The listing builds one solid part. Answer for the finished solid, in the listing's coordinates (mm). Coordinates: 2 decimals unless noted, no trailing zeros. Order: outer loops, then holes, each group sorted by start corner. A loop starts at its lowest first (then second) coordinate and runs counter-clockwise, first axis right, second up. Notation, with made-up numbers: (35.5, 72) -> (48.5, 72) arc R4 cw to (48.5, 77) -> close; hole circle Ø1 at (86.5, -5). An arc over 180 degrees is marked (long way). Return JSON: item names as keys, results as strings.
```python
from build123d import *

# Parameters (mm, degrees)
CYLINDER021_R          = 1.5
CYLINDER021_DEPTH      = 15
CYLINDER021_ROLL_ANGLE = 90
CYLINDER020_R          = 1.5
CYLINDER020_DEPTH      = 15
CYLINDER020_ROLL_ANGLE = 90
CYLINDER018_R          = 1.5
CYLINDER018_DEPTH      = 15
CYLINDER018_ROLL_ANGLE = 90
CYLINDER019_R          = 1.5
CYLINDER019_DEPTH      = 15
CYLINDER019_ROLL_ANGLE = 90
CYLINDER017_R          = 2
CYLINDER017_DEPTH      = 25
CYLINDER016_R          = 2
CYLINDER016_DEPTH      = 25
CYLINDER001_R          = 2
CYLINDER001_DEPTH      = 25
CYLINDER002_R          = 2
CYLINDER002_DEPTH      = 25
CYLINDER003_R          = 2
CYLINDER003_DEPTH      = 25
CYLINDER_R             = 2
CYLINDER_DEPTH         = 25
BOX_W                  = 50
BOX_H                  = 100
BOX_DEPTH              = 18
CYLINDER013_R          = 2
CYLINDER013_DEPTH      = 25
CYLINDER014_R          = 2
CYLINDER014_DEPTH      = 25
CYLINDER015_R          = 2
CYLINDER015_DEPTH      = 25
CYLINDER012_R          = 2
CYLINDER012_DEPTH      = 25
BOX002_W               = 50
BOX002_H               = 100
BOX002_DEPTH           = 18
CYLINDER009_R          = 2
CYLINDER009_DEPTH      = 25
CYLINDER010_R          = 2
CYLINDER010_DEPTH      = 25
CYLINDER011_R          = 2
CYLINDER011_DEPTH      = 25
CYLINDER008_R          = 2
CYLINDER008_DEPTH      = 25
BOX003_W               = 50
BOX003_H               = 100
BOX003_DEPTH           = 18
CYLINDER005_R          = 2
CYLINDER005_DEPTH      = 25
CYLINDER006_R          = 2
CYLINDER006_DEPTH      = 25
CYLINDER007_R          = 2
CYLINDER007_DEPTH      = 25
CYLINDER004_R          = 2
CYLINDER004_DEPTH      = 25
BOX001_W               = 50
BOX001_H               = 100
BOX001_DEPTH           = 18


with BuildPart() as cilindro019:
    # Cylinder021 → Cylinder021 (new body)
    with BuildSketch(Plane.XY):
        Circle(CYLINDER021_R)
    extrude(amount=CYLINDER021_DEPTH)


with BuildPart() as cilindro019_1:
    # Cylinder021 roll: moved
    add(cilindro019.part.rotate(Axis((0, 0, 0), (1, 0, 0)), CYLINDER021_ROLL_ANGLE))


with BuildPart() as cilindro019_2:
    # Cylinder021 placement: moved
    add(cilindro019_1.part.moved(Location((20, 15, 9))))


with BuildPart() as fusion006:
    # Cylinder020 → Cylinder020 (new body)
    with BuildSketch(Plane.XY):
        Circle(CYLINDER020_R)
    extrude(amount=CYLINDER020_DEPTH)


with BuildPart() as fusion006_1:
    # Cylinder020 roll: moved
    add(fusion006.part.rotate(Axis((0, 0, 0), (1, 0, 0)), CYLINDER020_ROLL_ANGLE))


with BuildPart() as fusion006_2:
    # Cylinder020 placement: moved
    add(fusion006_1.part.moved(Location((80, 15, 9))))

    # Fusion006: union Cilindro019
    add(cilindro019_2.part)


with BuildPart() as fusion006_3:
    # Fusion006 placement: moved
    add(fusion006_2.part.moved(Location((0, 0, 4))))


with BuildPart() as mirror_of_fusion006:
    # mirror001: instance of Fusion006
    add(fusion006_3.part.mirror(Plane(origin=(0, 100, 18), x_dir=(1, 0, 0), z_dir=(0, 1, 0))))


with BuildPart() as cilindro016:
    # Cylinder018 → Cylinder018 (new body)
    with BuildSketch(Plane.XY):
        Circle(CYLINDER018_R)
    extrude(amount=CYLINDER018_DEPTH)


with BuildPart() as cilindro016_1:
    # Cylinder018 roll: moved
    add(cilindro016.part.rotate(Axis((0, 0, 0), (1, 0, 0)), CYLINDER018_ROLL_ANGLE))


with BuildPart() as cilindro016_2:
    # Cylinder018 placement: moved
    add(cilindro016_1.part.moved(Location((20, 15, 9))))


with BuildPart() as fusion005:
    # Cylinder019 → Cylinder019 (new body)
    with BuildSketch(Plane.XY):
        Circle(CYLINDER019_R)
    extrude(amount=CYLINDER019_DEPTH)


with BuildPart() as fusion005_1:
    # Cylinder019 roll: moved
    add(fusion005.part.rotate(Axis((0, 0, 0), (1, 0, 0)), CYLINDER019_ROLL_ANGLE))


with BuildPart() as fusion005_2:
    # Cylinder019 placement: moved
    add(fusion005_1.part.moved(Location((80, 15, 9))))

    # Fusion005: union Cilindro016
    add(cilindro016_2.part)


with BuildPart() as fusion005_3:
    # Fusion005 placement: moved
    add(fusion005_2.part.moved(Location((0, 0, -4))))


with BuildPart() as mirror_of_fusion005:
    # mirror: instance of Fusion005
    add(fusion005_3.part.mirror(Plane(origin=(80, 100, 18), x_dir=(-1, 0, 0), z_dir=(0, -1, 0))))


with BuildPart() as huecocentral2:
    # Cylinder017 → Cylinder017 (new body)
    with BuildSketch(Plane(origin=(50, 119, 0), x_dir=(1, 0, 0), z_dir=(0, 0, 1))):
        Circle(CYLINDER017_R)
    extrude(amount=CYLINDER017_DEPTH)


with BuildPart() as huecocentral1:
    # Cylinder016 → Cylinder016 (new body)
    with BuildSketch(Plane(origin=(50, 81, 0), x_dir=(1, 0, 0), z_dir=(0, 0, 1))):
        Circle(CYLINDER016_R)
    extrude(amount=CYLINDER016_DEPTH)


with BuildPart() as cilindro001:
    # Cylinder001 → Cylinder001 (new body)
    with BuildSketch(Plane(origin=(11, 72, 0), x_dir=(1, 0, 0), z_dir=(0, 0, 1))):
        Circle(CYLINDER001_R)
    extrude(amount=CYLINDER001_DEPTH)


with BuildPart() as cilindro002:
    # Cylinder002 → Cylinder002 (new body)
    with BuildSketch(Plane(origin=(29, 48, 0), x_dir=(1, 0, 0), z_dir=(0, 0, 1))):
        Circle(CYLINDER002_R)
    extrude(amount=CYLINDER002_DEPTH)


with BuildPart() as cilindro003:
    # Cylinder003 → Cylinder003 (new body)
    with BuildSketch(Plane(origin=(29, 72, 0), x_dir=(1, 0, 0), z_dir=(0, 0, 1))):
        Circle(CYLINDER003_R)
    extrude(amount=CYLINDER003_DEPTH)


with BuildPart() as huecos:
    # Cylinder → Cylinder (new body)
    with BuildSketch(Plane(origin=(11, 48, 0), x_dir=(1, 0, 0), z_dir=(0, 0, 1))):
        Circle(CYLINDER_R)
    extrude(amount=CYLINDER_DEPTH)

    # Fusion: union Cilindro001, Cilindro002, Cilindro003
    add(cilindro001.part)
    add(cilindro002.part)
    add(cilindro003.part)


with BuildPart() as cut003:
    # Box → Box (new body)
    with BuildSketch(Plane.XY):
        with Locations((25, 50)):
            Rectangle(BOX_W, BOX_H)
    extrude(amount=BOX_DEPTH)

    # Cut003: cut Huecos
    add(huecos.part, mode=Mode.SUBTRACT)


with BuildPart() as cilindro013:
    # Cylinder013 → Cylinder013 (new body)
    with BuildSketch(Plane(origin=(11, 72, 0), x_dir=(1, 0, 0), z_dir=(0, 0, 1))):
        Circle(CYLINDER013_R)
    extrude(amount=CYLINDER013_DEPTH)


with BuildPart() as cilindro014:
    # Cylinder014 → Cylinder014 (new body)
    with BuildSketch(Plane(origin=(29, 48, 0), x_dir=(1, 0, 0), z_dir=(0, 0, 1))):
        Circle(CYLINDER014_R)
    extrude(amount=CYLINDER014_DEPTH)


with BuildPart() as cilindro015:
    # Cylinder015 → Cylinder015 (new body)
    with BuildSketch(Plane(origin=(29, 72, 0), x_dir=(1, 0, 0), z_dir=(0, 0, 1))):
        Circle(CYLINDER015_R)
    extrude(amount=CYLINDER015_DEPTH)


with BuildPart() as huecos003:
    # Cylinder012 → Cylinder012 (new body)
    with BuildSketch(Plane(origin=(11, 48, 0), x_dir=(1, 0, 0), z_dir=(0, 0, 1))):
        Circle(CYLINDER012_R)
    extrude(amount=CYLINDER012_DEPTH)

    # Fusion003: union Cilindro013, Cilindro014, Cilindro015
    add(cilindro013.part)
    add(cilindro014.part)
    add(cilindro015.part)


with BuildPart() as huecos003_1:
    # Fusion003 placement: moved
    add(huecos003.part.moved(Location((0, 80, 0))))


with BuildPart() as cut:
    # Box002 → Box002 (new body)
    with BuildSketch(Plane(origin=(0, 100, 0), x_dir=(1, 0, 0), z_dir=(0, 0, 1))):
        with Locations((25, 50)):
            Rectangle(BOX002_W, BOX002_H)
    extrude(amount=BOX002_DEPTH)

    # Cut: cut Huecos003
    add(huecos003_1.part, mode=Mode.SUBTRACT)


with BuildPart() as cilindro009:
    # Cylinder009 → Cylinder009 (new body)
    with BuildSketch(Plane(origin=(11, 72, 0), x_dir=(1, 0, 0), z_dir=(0, 0, 1))):
        Circle(CYLINDER009_R)
    extrude(amount=CYLINDER009_DEPTH)


with BuildPart() as cilindro010:
    # Cylinder010 → Cylinder010 (new body)
    with BuildSketch(Plane(origin=(29, 48, 0), x_dir=(1, 0, 0), z_dir=(0, 0, 1))):
        Circle(CYLINDER010_R)
    extrude(amount=CYLINDER010_DEPTH)


with BuildPart() as cilindro011:
    # Cylinder011 → Cylinder011 (new body)
    with BuildSketch(Plane(origin=(29, 72, 0), x_dir=(1, 0, 0), z_dir=(0, 0, 1))):
        Circle(CYLINDER011_R)
    extrude(amount=CYLINDER011_DEPTH)


with BuildPart() as huecos002:
    # Cylinder008 → Cylinder008 (new body)
    with BuildSketch(Plane(origin=(11, 48, 0), x_dir=(1, 0, 0), z_dir=(0, 0, 1))):
        Circle(CYLINDER008_R)
    extrude(amount=CYLINDER008_DEPTH)

    # Fusion002: union Cilindro009, Cilindro010, Cilindro011
    add(cilindro009.part)
    add(cilindro010.part)
    add(cilindro011.part)


with BuildPart() as huecos002_1:
    # Fusion002 placement: moved
    add(huecos002.part.moved(Location((-40, 80, 0))))


with BuildPart() as cut001:
    # Box003 → Box003 (new body)
    with BuildSketch(Plane(origin=(-50, 100, 0), x_dir=(1, 0, 0), z_dir=(0, 0, 1))):
        with Locations((25, 50)):
            Rectangle(BOX003_W, BOX003_H)
    extrude(amount=BOX003_DEPTH)

    # Cut001: cut Huecos002
    add(huecos002_1.part, mode=Mode.SUBTRACT)


with BuildPart() as cut001_1:
    # Cut001 placement: moved
    add(cut001.part.moved(Location((100, 0, 0))))


with BuildPart() as cilindro005:
    # Cylinder005 → Cylinder005 (new body)
    with BuildSketch(Plane(origin=(11, 72, 0), x_dir=(1, 0, 0), z_dir=(0, 0, 1))):
        Circle(CYLINDER005_R)
    extrude(amount=CYLINDER005_DEPTH)


with BuildPart() as cilindro006:
    # Cylinder006 → Cylinder006 (new body)
    with BuildSketch(Plane(origin=(29, 48, 0), x_dir=(1, 0, 0), z_dir=(0, 0, 1))):
        Circle(CYLINDER006_R)
    extrude(amount=CYLINDER006_DEPTH)


with BuildPart() as cilindro007:
    # Cylinder007 → Cylinder007 (new body)
    with BuildSketch(Plane(origin=(29, 72, 0), x_dir=(1, 0, 0), z_dir=(0, 0, 1))):
        Circle(CYLINDER007_R)
    extrude(amount=CYLINDER007_DEPTH)


with BuildPart() as huecos001:
    # Cylinder004 → Cylinder004 (new body)
    with BuildSketch(Plane(origin=(11, 48, 0), x_dir=(1, 0, 0), z_dir=(0, 0, 1))):
        Circle(CYLINDER004_R)
    extrude(amount=CYLINDER004_DEPTH)

    # Fusion001: union Cilindro005, Cilindro006, Cilindro007
    add(cilindro005.part)
    add(cilindro006.part)
    add(cilindro007.part)


with BuildPart() as huecos001_1:
    # Fusion001 placement: moved
    add(huecos001.part.moved(Location((-40, 0, 0))))


with BuildPart() as cut009:
    # Box001 → Box001 (new body)
    with BuildSketch(Plane(origin=(-50, 0, 0), x_dir=(1, 0, 0), z_dir=(0, 0, 1))):
        with Locations((25, 50)):
            Rectangle(BOX001_W, BOX001_H)
    extrude(amount=BOX001_DEPTH)

    # Cut002: cut Huecos001
    add(huecos001_1.part, mode=Mode.SUBTRACT)


with BuildPart() as cut009_1:
    # Cut002 placement: moved
    add(cut009.part.moved(Location((100, 0, 0))))

    # Fusion004: union Cut003, Cut, Cut001
    add(cut003.part)
    add(cut.part)
    add(cut001_1.part)

    # Cut004: cut HuecoCentral1
    add(huecocentral1.part, mode=Mode.SUBTRACT)

    # Cut005: cut HuecoCentral2
    add(huecocentral2.part, mode=Mode.SUBTRACT)

    # Cut006: cut Mirror of Fusion005
    add(mirror_of_fusion005.part, mode=Mode.SUBTRACT)

    # Cut007: cut Fusion005
    add(fusion005_3.part, mode=Mode.SUBTRACT)

    # Cut008: cut Fusion006
    add(fusion006_3.part, mode=Mode.SUBTRACT)

    # Cut009: cut Mirror of Fusion006
    add(mirror_of_fusion006.part, mode=Mode.SUBTRACT)


solid = cut009_1.part
```
Item 1: Flat-ended cylindrical pins translate along their axes: pin 1 (1.5 mm diameter, centred on x = 80.5, z = 5.5, fed in from +Y); pin 2 (2.5 mm diameter, centred on x = 20, z = 13, fed in from -Y). Find the tip coordinate at first contact, or state that the pin passes through.
Answer list:
{"pin 1": "y = 185", "pin 2": "y = 15"}
Item 2: Determine the mould class of faces 1 (the flat face through (49, 101, 0)), 2 (the cylindrical face through (51.075, 120.686, 8.874)), 3 (the flat face through (0, 99, 9)), 4 (the cylindrical face through (89.923, 126.226, 8.874)) for opening direction X: pulls with the +X half, pulls with the -X half, needs draft (parallel to the pull), parting line crosses it, or undercut.
Answer list:
{"face 1": "needs draft", "face 2": "undercut", "face 3": "pulls with the -X half", "face 4": "undercut"}
Item 3: The part is cut by section C-C on x = 50. Determine the outline of the cut face in (y, z).
Answer list:
{"outline": "(0, 0) -> (79, 0) -> (79, 18) -> (0, 18) -> close; (83, 0) -> (117, 0) -> (117, 18) -> (83, 18) -> close; (121, 0) -> (200, 0) -> (200, 18) -> (121, 18) -> close"}
Item 4: Find the intervals of material crossed by probe 1 along Y at (x, z) = (11, 8); probe 2 along Z at (x, y) = (20, 3.25); probe 3 along X at (y, z) = (152, 5.25), in increasing order.
Answer list:
{"probe 1": "0 to 46, 50 to 70, 74 to 126, 130 to 150, 154 to 200", "probe 2": "0 to 3.5, 6.5 to 11.5, 14.5 to 18", "probe 3": "0 to 9, 13 to 27, 31 to 69, 73 to 87, 91 to 100"}
Item 5: The part is cut by section A-A on y = 119. Determine the outline of the cut face in (x, z), plus the area to 3 significant figures.
Answer list:
{"outline": "(0, 0) -> (48, 0) -> (48, 18) -> (0, 18) -> close; (52, 0) -> (100, 0) -> (100, 18) -> (52, 18) -> close", "area": "1,730 mm2"}
Item 6: The part is cut by section B-B on x = 29. Determine the outline of the cut face in (y, z), plus the area to 3 significant figures.
Answer list:
{"outline": "(0, 0) -> (46, 0) -> (46, 18) -> (0, 18) -> close; (50, 0) -> (70, 0) -> (70, 18) -> (50, 18) -> close; (74, 0) -> (126, 0) -> (126, 18) -> (74, 18) -> close; (130, 0) -> (150, 0) -> (150, 18) -> (130, 18) -> close; (154, 0) -> (200, 0) -> (200, 18) -> (154, 18) -> close", "area": "3,310 mm2"}
Item 7: The part is cut by section D-D on y = 152. Determine the outline of the cut face in (x, z).
Answer list:
{"outline": "(0, 0) -> (9, 0) -> (9, 18) -> (0, 18) -> close; (13, 0) -> (27, 0) -> (27, 18) -> (13, 18) -> close; (31, 0) -> (69, 0) -> (69, 18) -> (31, 18) -> close; (73, 0) -> (87, 0) -> (87, 18) -> (73, 18) -> close; (91, 0) -> (100, 0) -> (100, 18) -> (91, 18) -> close"}
